```python
from build123d import *

# Parameters (mm, degrees)
CROQUIS1_R              = 25
CROQUIS1_W              = 10.2
CROQUIS1_H              = 10.2
SALIENTE_EXTRUIR1_DEPTH = 5
CROQUIS2_R              = 3.5
CORTAR_EXTRUIR1_DEPTH   = 47


with BuildPart() as part:
    # Croquis1 → Saliente-Extruir1 (new body)
    with BuildSketch(Plane(origin=(0, 0, 0), x_dir=(1, 0, 0), z_dir=(0, 1, 0))):
        Circle(CROQUIS1_R)
        with Locations((-15, 0)):
            Rectangle(CROQUIS1_W, CROQUIS1_H, mode=Mode.SUBTRACT)
        with Locations((15, 0)):
            Rectangle(CROQUIS1_W, CROQUIS1_H, mode=Mode.SUBTRACT)
        with Locations((0, 15)):
            Rectangle(CROQUIS1_W, CROQUIS1_H, mode=Mode.SUBTRACT)
        with Locations((0, -15)):
            Rectangle(CROQUIS1_W, CROQUIS1_H, mode=Mode.SUBTRACT)
    extrude(amount=SALIENTE_EXTRUIR1_DEPTH)

    # Croquis2 → Cortar-Extruir1 (cut)
    with BuildSketch(Plane(origin=(0, 5, 0), x_dir=(1, 0, 0), z_dir=(0, 1, 0))):
        Circle(CROQUIS2_R)
    extrude(amount=-CORTAR_EXTRUIR1_DEPTH, mode=Mode.SUBTRACT)


solid = part.part
```
Geometry check sheet. Reference: the model listing, model coordinates, mm. A direction names the side the tool comes from. Coordinates: 2 decimals unless noted, no trailing zeros. Loops run counter-clockwise (first coordinate to the right, second up) from the corner with the lowest first, then second, coordinate; pieces in that order, holes last.
Item 1: Sectioned sample at B-B, the plane z = 0. Record the boundary of the cut face in (x, y).
Item 2: Thickness scan on line 1 (Z direction, x = 0, y = 1.5); line 2 (Z direction, x = -1.5, y = 2.5). Record the ranges inside material, lowest first.
Item 3: Access from +Z, -Z, +X, -X, +Y, -Y to the whole of each face (thin tool, end or side, straight path). Record for faces 5 (the face through (0, 2, -20.1)), 6 (the face through (0, 5, 5)).
Item 4: Release check for a two-part mould opening along X. For faces 1 (the face through (20.1, 2, 0)), 2 (the face through (-5.1, 2, 15)), 3 (the face through (0, 0, 5)), 4 (the face through (23.846, 2.465, -7.509)) record: released by +X, released by -X, zero draft, split by the parting line, or undercut.
Item 5: Go/stop test with flat-tipped pins: pin 1 Ø2 at (y, z) = (3, 0.5) entering from +X; pin 2 Ø2.5 at (x, y) = (13, 2) entering from +Z; pin 3 Ø2.5 at (y, z) = (2.5, 16.5) entering from +X; pin 4 Ø1.5 at (x, y) = (9.5, 1.5) entering from -Z. Record where each tip stops, or that it passes through.
Item 6: Sectioned sample at A-A, the plane y = 3.75. Record the boundary of the cut face in (x, z).
Item 7: Sectioned sample at D-D, the plane x = -18. Record the boundary of the cut face in (y, z), then the cut area to 3 significant figures.
Item 8: Sectioned sample at C-C, the plane x = 0. Record the boundary of the cut face in (y, z).
Check result:
1. outline: (-25, 0) - (-20.1, 0) - (-20.1, 5) - (-25, 5) - close; (-9.9, 0) - (-3.5, 0) - (-3.5, 5) - (-9.9, 5) - close; (3.5, 0) - (9.9, 0) - (9.9, 5) - (3.5, 5) - close; (20.1, 0) - (25, 0) - (25, 5) - (20.1, 5) - close
2. line 1: z = -25 to -20.1, -9.9 to -3.5, 3.5 to 9.9, 20.1 to 25
2. line 2: z = -24.95 to -20.1, -9.9 to -3.16, 3.16 to 9.9, 20.1 to 24.95
3. face 5: +Y, -Y
3. face 6: +Z, -Z, +X, -X, +Y
4. face 1: undercut
4. face 2: undercut
4. face 3: zero draft
4. face 4: split by the parting line
5. pin 1: stops at x = 25
5. pin 2: stops at z = 22.07
5. pin 3: stops at x = 19.81
5. pin 4: stops at z = -23.42
6. outline: circle Ø50 at (0, 0); hole (-20.1, -5.1) - (-9.9, -5.1) - (-9.9, 5.1) - (-20.1, 5.1) - close; hole (-5.1, -20.1) - (5.1, -20.1) - (5.1, -9.9) - (-5.1, -9.9) - close; hole (-5.1, 9.9) - (5.1, 9.9) - (5.1, 20.1) - (-5.1, 20.1) - close; hole circle Ø7 at (0, 0); hole (9.9, -5.1) - (20.1, -5.1) - (20.1, 5.1) - (9.9, 5.1) - close
7. outline: (0, -17.35) - (5, -17.35) - (5, -5.1) - (0, -5.1) - close; (0, 5.1) - (5, 5.1) - (5, 17.35) - (0, 17.35) - close
7. area: 122 mm2
8. outline: (0, -25) - (5, -25) - (5, -20.1) - (0, -20.1) - close; (0, -9.9) - (5, -9.9) - (5, -3.5) - (0, -3.5) - close; (0, 3.5) - (5, 3.5) - (5, 9.9) - (0, 9.9) - close; (0, 20.1) - (5, 20.1) - (5, 25) - (0, 25) - close
